from build123d import *

# Parameters (mm, degrees)
F0_R     = 46.5
F1_DEPTH = 23
F3_DEPTH = 15
F4_R     = 1
F5_R     = 45
F5_R_2   = 44
F6_DEPTH = 20
F7_R     = 0.5
F8_R     = 2


# Not quite as in the source:
# - a feature names something its author has since deleted; it is built from what else it names


with BuildPart() as f1:
    # F0 (on Top) → F1 (new body)
    with BuildSketch(Plane.XY):
        Circle(F0_R)
        with BuildLine():
            ThreePointArc((-15.375, -38.0080172464), (-41, 0), (-15.375, 38.0080172464))
            ThreePointArc((-15.375, 38.0080172464), (-6.9688470506, 37.1271997267), (-3, 29.6647939484))
            Line((-3, 29.6647939484), (-3, -29.6647939484))
            ThreePointArc((-3, -29.6647939484), (-6.9688470506, -37.1271997267), (-15.375, -38.0080172464))
        make_face(mode=Mode.SUBTRACT)
        with BuildLine():
            Line((3, -29.6647939484), (3, 29.6647939484))
            ThreePointArc((3, 29.6647939484), (6.9688470506, 37.1271997267), (15.375, 38.0080172464))
            ThreePointArc((15.375, 38.0080172464), (41, 0), (15.375, -38.0080172464))
            ThreePointArc((15.375, -38.0080172464), (6.9688470506, -37.1271997267), (3, -29.6647939484))
        make_face(mode=Mode.SUBTRACT)
    extrude(amount=-F1_DEPTH)

    # F2 (on face) → F3 (cut)
    with BuildSketch(Plane(origin=(0, 0, -23), x_dir=(1, 0, 0), z_dir=(0, 0, -1))):
        with BuildLine():
            ThreePointArc((-15.75, -38.9350420573), (-6.4098300563, -37.9563559243), (-2, -29.6647939484))
            Line((-2, -29.6647939484), (-2, 29.6647939484))
            ThreePointArc((-2, 29.6647939484), (-6.4098300563, 37.9563559243), (-15.75, 38.9350420573))
            ThreePointArc((-15.75, 38.9350420573), (-42, 0), (-15.75, -38.9350420573))
        make_face()
        with BuildLine():
            Line((-3, 29.6647939484), (-3, -29.6647939484))
            ThreePointArc((-3, -29.6647939484), (-6.9688470506, -37.1271997267), (-15.375, -38.0080172464))
            ThreePointArc((-15.375, -38.0080172464), (-41, 0), (-15.375, 38.0080172464))
            ThreePointArc((-15.375, 38.0080172464), (-6.9688470506, 37.1271997267), (-3, 29.6647939484))
        make_face(mode=Mode.SUBTRACT)
        with BuildLine():
            ThreePointArc((2, -29.6647939484), (6.4098300563, -37.9563559243), (15.75, -38.9350420573))
            ThreePointArc((15.75, -38.9350420573), (42, 0), (15.75, 38.9350420573))
            ThreePointArc((15.75, 38.9350420573), (6.4098300563, 37.9563559243), (2, 29.6647939484))
            Line((2, 29.6647939484), (2, -29.6647939484))
        make_face()
        with BuildLine():
            ThreePointArc((3, 29.6647939484), (6.9688470506, 37.1271997267), (15.375, 38.0080172464))
            ThreePointArc((15.375, 38.0080172464), (41, 0), (15.375, -38.0080172464))
            ThreePointArc((15.375, -38.0080172464), (6.9688470506, -37.1271997267), (3, -29.6647939484))
            Line((3, -29.6647939484), (3, 29.6647939484))
        make_face(mode=Mode.SUBTRACT)
    extrude(amount=-F3_DEPTH, mode=Mode.SUBTRACT)

    # F4
    f4_edges = [f1.edges().sort_by_distance(p)[0] for p in [
        (-41, 0, 0),
        (3, 0, 0),
    ]]
    fillet(f4_edges, radius=F4_R)

    # F5 (on face) → F6 (cut)
    with BuildSketch(Plane(origin=(0, 0, -23), x_dir=(1, 0, 0), z_dir=(0, 0, -1))):
        Circle(F5_R)
        Circle(F5_R_2, mode=Mode.SUBTRACT)
    extrude(amount=-F6_DEPTH, mode=Mode.SUBTRACT)

    # F7
    f7_edges = [f1.edges().sort_by_distance(p)[0] for p in [
        (-44, 0, -23),
        (-46.5, 0, -23),
    ]]
    fillet(f7_edges, radius=F7_R)

    # F8
    f8_edges = [f1.edges().sort_by_distance(p)[0] for p in [
        (-46.5, 0, 0),
    ]]
    fillet(f8_edges, radius=F8_R)


solid = f1.part
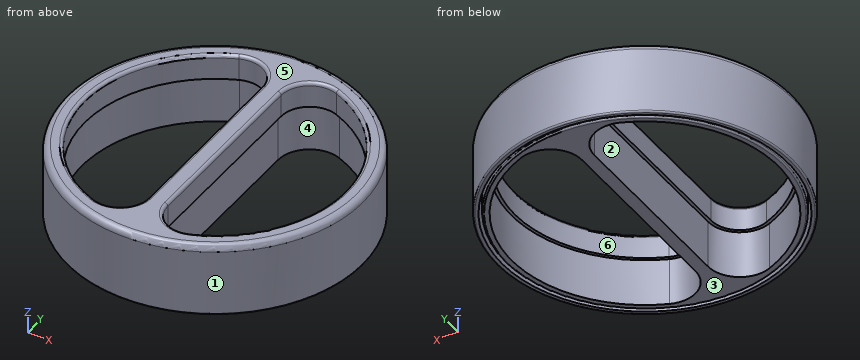
The listing builds one solid part. Answer for the finished solid, in the listing's coordinates (mm). Face numbers are marked on the shaded views. A direction names the side the tool comes from. Give positions to 0.01 mm unless a question says otherwise; leave off trailing zeros. Order: outer loops, then holes, each group sorted by start corner. A loop starts at its lowest first (then second) coordinate and runs counter-clockwise, first axis right, second up. Notation, with made-up numbers: (77, -25) - (131, -25) arc R24 cw to (131, 13) - close; hole circle Ø8 at (58, -28.75). An arc over 180 degrees is marked (long way). One line per item, written item: value. Start each with the question number.
1) A tool of negligible diameter and unlimited length cuts with its end or side. For the marked faces 4, 5 and 6, from which of +Z, -Z, +X, -X, +Y, -Y can it reach the whole face along a straight path? Write none if from no direction.
2) Find the intervals of material crossed by L1, parallel to Y at x = 0, z = -9.75; L2, parallel to X at y = 3.5, z = -18.25; L3, parallel to Y at x = 37.5, z = -14.25, in increasing order.
3) A cutting plane is placed at A-A on z = -20. Give the vertices of the cut face in (x, y), then the cut area to 3 significant figures.
4) A cutting plane is placed at C-C on y = 0. State how many separate pieces and enclosed holes the cut face has, then the cut area to 3 significant figures.
5) A cutting plane is placed at B-B on x = 0. Give the vertices of the cut face in (y, z), then the cut area to 3 significant figures.
6) Given pin 1 Ø3.5 at (y, z) = (13, -4) entering from +X; pin 2 Ø1 at (x, z) = (9.5, -10.5) entering from -Y; pin 3 Ø3 at (x, z) = (-29, -12) entering from -Y, each flat-ended and moving along its own axis, determine where each tip first touches the part or whether it passes through.
7) The mould has two halves that part along Y. Classify the marked faces 1, 2 and 3: released by +Y, released by -Y, zero draft, split by the parting line, or undercut.
Answer sheet:
1. face 4: -Z
1. face 5: +Z, +X, -X, +Y, -Y
1. face 6: +Z, -Z
2. L1: y = -46.5 to -45, -44 to 44, 45 to 46.5
2. L2: x = -46.37 to -44.86, -43.86 to -41.85, -2 to 2, 41.85 to 43.86, 44.86 to 46.37
2. L3: y = -27.5 to -24.87, -23.02 to -18.91, 18.91 to 23.02, 24.87 to 27.5
3. outline: circle Ø93 at (0, 0); circle Ø88 at (0, 0); hole circle Ø90 at (0, 0); hole (-15.75, -38.94) arc R10 ccw to (-2, -29.66) - (-2, 29.66) arc R10 ccw to (-15.75, 38.94) arc R42 ccw to start; hole (2, -29.66) arc R10 ccw to (15.75, -38.94) arc R42 ccw to (15.75, 38.94) arc R10 ccw to (2, 29.66) - close
3. area: 1,460 mm2
4. separate pieces: 3
4. enclosed holes: 0
4. area: 288 mm2
5. outline: (-46.5, -22.5) arc R0.5 ccw to (-46, -23) - (-45, -23) - (-45, -3) - (-44, -3) - (-44, -22.5) arc R0.5 ccw to (-43.5, -23) - (43.5, -23) arc R0.5 ccw to (44, -22.5) - (44, -3) - (45, -3) - (45, -23) - (46, -23) arc R0.5 ccw to (46.5, -22.5) - (46.5, -2) arc R2 ccw to (44.5, 0) - (-44.5, 0) arc R2 ccw to (-46.5, -2) - close
5. area: 2,100 mm2
6. pin 1: stops at x = 45.12
6. pin 2: stops at y = -45.62
6. pin 3: stops at y = -37.5
7. face 1: split by the parting line
7. face 2: undercut
7. face 3: zero draft
